```python
from build123d import *

# Parameters (mm, degrees)
SKETCH_R           = 20
SKETCH_R_2         = 8.5
PAD_DEPTH          = 15
SKETCH001_R        = 17
SKETCH001_R_2      = 11.5
POCKET_DEPTH       = 12.001
SKETCH002_W        = 3
SKETCH002_H        = 8.150041
PAD001_DEPTH       = 6
POLARPATTERN_COUNT = 5
SKETCH003_R        = 11.5
POCKET001_DEPTH    = 4.001


with BuildPart() as part:
    # Sketch → Pad (new body)
    with BuildSketch(Plane.XZ):
        Circle(SKETCH_R)
        Circle(SKETCH_R_2, mode=Mode.SUBTRACT)
    extrude(amount=PAD_DEPTH)

    # Sketch001 → Pocket (cut, through all)
    with BuildSketch(Plane.XZ.offset(3)):
        Circle(SKETCH001_R)
        Circle(SKETCH001_R_2, mode=Mode.SUBTRACT)
    extrude(amount=POCKET_DEPTH, mode=Mode.SUBTRACT)

    # Sketch002 → Pad001 (join)
    with BuildSketch(Plane.XZ.offset(3)):
        with Locations((0, 14.096249)):
            Rectangle(SKETCH002_W, SKETCH002_H)
    pad001 = extrude(amount=PAD001_DEPTH)

    # PolarPattern: Pad001 ×5 about axis
    polarpattern_axis = Axis((0, -3, 0), (0, -1, 0))
    for i in range(1, POLARPATTERN_COUNT):
        add(pad001.rotate(polarpattern_axis, i * 360 / POLARPATTERN_COUNT))

    # Sketch003 → Pocket001 (cut, through all)
    with BuildSketch(Plane.XZ.offset(11)):
        Circle(SKETCH003_R)
    extrude(amount=POCKET001_DEPTH, mode=Mode.SUBTRACT)


solid = part.part
```
Check sheet for the modelled part. Datum: model origin and axes. Units: mm. A direction names the side the tool comes from. Give positions to 0.01 mm unless a question says otherwise; leave off trailing zeros. Loops run counter-clockwise (first coordinate to the right, second up) from the corner with the lowest first, then second, coordinate; pieces in that order, holes last. Notation, with made-up numbers: M 50,-39.5 L 100,-39.5 A20 cw 100,-12.5 Z; hole C 67.25,-13.75 d8. An arc over 180 degrees is marked long. Answer in a Markdown table with one row per item.
1) Mould release check, pull along Z, two halves, no side actions. Record for faces 1 (the face through (0, 0, -9)), 2 (the face through (8, -9, -12)): released by +Z, released by -Z, zero draft, split by the parting line, or undercut.
Solutions:
| item | result |
|---|---|
| face 1 | zero draft |
| face 2 | undercut |
2) Tool access check on faces 3 (the face through (-16.984, -8.916, 0.747)), 4 (the face through (-9, -15, -15)). Record the directions out of +Z, -Z, +X, -X, +Y, -Y that give a thin tool (end or side, any length) a straight path to the whole face; none if there is none.
Solutions:
| item | result |
|---|---|
| face 3 | -Y |
| face 4 | +Z, -Z, +X, -X, -Y |
3) Depth check by flat-ended pin: pin 1 (6 mm diameter, centred on x = 7.5, z = -12.5, fed in from -Y); pin 2 (1 mm diameter, centred on x = 9, y = -7, fed in from -Z); pin 3 (4 mm diameter, centred on x = -10, y = -9.5, fed in from -Z); pin 4 (5 mm diameter, centred on y = -8, z = -8.5, fed in from -X). Enter the tip coordinate at first touch or a pass-through.
Solutions:
| item | result |
|---|---|
| pin 1 | stops at y = -15 |
| pin 2 | stops at z = -18.1 |
| pin 3 | stops at z = -18.33 |
| pin 4 | stops at x = -19.08 |
4) Cross-section at C-C (y = -9.75). Enter the section's corners in (x, z).
Solutions:
| item | result |
|---|---|
| outline | C 0,0 d40; C 0,0 d23; hole C 0,0 d34; hole C 0,0 d17 |
5) Cross-section at B-B (x = -1). Enter the section's corners in (y, z).
Solutions:
| item | result |
|---|---|
| outline | M -15,-19.97 L 0,-19.97 L 0,-8.44 L -11,-8.44 L -11,-11.46 L -3,-11.46 L -3,-16.97 L -15,-16.97 Z; M -15,16.97 L -9,16.97 L -9,11.46 L -11,11.46 L -11,8.44 L 0,8.44 L 0,19.97 L -15,19.97 Z |
6) Cross-section at A-A (z = 0). Enter the section's corners in (x, y), plus the area to 3 significant figures.
Solutions:
| item | result |
|---|---|
| outline | M -20,-15 L -17,-15 L -17,-3 L -11.5,-3 L -11.5,-11 L -8.5,-11 L -8.5,0 L -20,0 Z; M 8.5,-11 L 11.5,-11 L 11.5,-3 L 17,-3 L 17,-15 L 20,-15 L 20,0 L 8.5,0 Z |
| area | 189 mm^2 |
7) Cross-section at D-D (y = -2.25). Enter the section's corners in (x, z).
Solutions:
| item | result |
|---|---|
| outline | C 0,0 d40; hole C 0,0 d17 |
8) Thickness scan on line 1 (Z direction, x = 0, y = -6.5); line 2 (Z direction, x = 0, y = -10.5); line 3 (X direction, y = -5, z = -4). Record the ranges inside material, lowest first.
Solutions:
| item | result |
|---|---|
| line 1 | z = -20 to -17, -11.5 to -8.5, 8.5 to 20 |
| line 2 | z = -20 to -17, -11.5 to -8.5, 8.5 to 11.5, 17 to 20 |
| line 3 | x = -19.6 to -16.52, -10.78 to -7.5, 7.5 to 10.78, 16.52 to 19.6 |
